Part model, mm, in its own coordinate system. A direction names the side the tool comes from. Give positions to 0.01 mm unless a question says otherwise; leave off trailing zeros. Write each loop counter-clockwise with the first axis right and the second up, starting at its lowest first coordinate (ties: lowest second). Pieces come first, ordered by that corner, then holes.
Autodesk Inventor part; units mm, degrees
ref_plane "YZ Plane" through (0, 0, 0) normal (1, 0, 0) x (0, 1, 0)
ref_plane "XZ Plane" through (0, 0, 0) normal (0, 1, 0) x (-1, 0, 0)
ref_plane "XY Plane" through (0, 0, 0) normal (0, 0, 1) x (1, 0, 0)
sketch "Sketch1" plane through (0, 0, 0) normal (0, 0, 1) x (1, 0, 0)
  line L0 (0, 0) -> (40, 0)
  line L1 (40, 0) -> (40, -40.5)
  line L2 (40, -40.5) -> (0, -40.5)
  line L3 (0, -40.5) -> (0, 0)
  dimension "d0" = 40
  dimension "d1" = 40.5
extrude "Extrusion1" add sketch "Sketch1" along normal mid plane 20
sketch "Sketch2" plane through (0, -40.5, 10) normal (-1, 0, 0) x (0, 0, 1)
  line L0 (0, 0) -> (-20, 0)
  line L1 (-20, 0) -> (-20, 40.5)
  line L2 (0, 40.5) -> (0, 0)
  circle A0 centre (-10, 10) radius 6
  line L3 (-20, 20.25) -> (0, 20.25)
  circle A1 centre (-10, 30.5) radius 6
  point P0 (-10, 40.5)
  dimension "d4" = 12
  dimension "d5" = 10
  dimension "d6" = 10
extrude "Extrusion2" add sketch "Sketch2" along normal blind 1.5 contours A0
sketch "Sketch3" plane through (40, -40.5, 10) normal (1, 0, 0) x (0, 0, -1)
  circle A0 centre (10, 10) radius 6
  circle A1 centre (10, 10) radius 6
  line L0 (0, 40.5) -> (0, 0)
  line L1 (0, 20.25) -> (20, 20.25)
  line L2 (20, 0) -> (20, 40.5)
  circle A2 centre (10, 30.5) radius 6
  point P0 (10, 40.5)
extrude "Extrusion4" add sketch "Sketch3" along normal blind 1.5 contours A0
extrude "Extrusion5" add sketch "Sketch2" along normal blind 0.1 contours A1
extrude "Extrusion6" add sketch "Sketch3" along normal blind 0.1 contours A2
properties part number "Motor"
1) Saw through at D-D (z = 8.75). Write the cut outline in (x, y), and give its area (3 significant figures).
Check result:
outline: (0, -40.5) - (40, -40.5) - (40, 0) - (0, 0) - close
area: 1,620 mm2
2) 3-axis set-ups, long thin cutter, end or side, ignore diameter. For faces 4 (the flat face through (41.5, -30, 0)), 5 (the cylindrical face through (40.74, -24.643, 1.301)), 6 (the flat face through (-0.1, -10, 0)), 7 (the flat face through (0, -21, 0)), 8 (the flat face through (20, -20, -10)): which of +Z, -Z, +X, -X, +Y, -Y reach the whole face in a straight line?
Check result:
face 4: +Z, -Z, +X, +Y, -Y
face 5: +X
face 6: +Z, -Z, -X, +Y
face 7: -X
face 8: -Z, +X, -X, +Y, -Y
3) Flat gauge pin, fed straight in: P1, Ø9.5, axis at y = -8.5, z = 2, coming from the -X side. Where does the tip first touch, or does it go through?
Check result:
P1: stops at x = -0.1
4) Saw through at B-B (z = 0). Write the cut outline in (x, y), and give its area (3 significant figures).
Check result:
outline: (-1.5, -36.5) - (0, -36.5) - (0, -40.5) - (40, -40.5) - (40, -36.5) - (41.5, -36.5) - (41.5, -24.5) - (40, -24.5) - (40, -16) - (40.1, -16) - (40.1, -4) - (40, -4) - (40, 0) - (0, 0) - (0, -4) - (-0.1, -4) - (-0.1, -16) - (0, -16) - (0, -24.5) - (-1.5, -24.5) - close
area: 1,660 mm2
5) Saw through at C-C (y = -10). Write the cut outline in (x, z).
Check result:
outline: (-0.1, -6) - (0, -6) - (0, -10) - (40, -10) - (40, -6) - (40.1, -6) - (40.1, 6) - (40, 6) - (40, 10) - (0, 10) - (0, 6) - (-0.1, 6) - close
6) Drill centre lines: L1, parallel to X at y = -9.5, z = 6.75; L2, parallel to X at y = -7, z = 2. Where is each one in solid material? Low to high.
Check result:
L1: x = 0 to 40
L2: x = -0.1 to 40.1
7) Mould opens along Y. For faces 1 (the flat face through (40, -20, 0)), 2 (the flat face through (40.1, -10, 0)), 3 (the flat face through (20, 0, 0)) say: +Y half, -Y half, draft (parallel to the pull), parting line (faces both ways), or undercut.
Check result:
face 1: undercut
face 2: draft
face 3: +Y half
8) Saw through at A-A (y = -30.5). Write the cut outline in (x, z), and give its area (3 significant figures).
Check result:
outline: (-1.5, -6) - (0, -6) - (0, -10) - (40, -10) - (40, -6) - (41.5, -6) - (41.5, 6) - (40, 6) - (40, 10) - (0, 10) - (0, 6) - (-1.5, 6) - close
area: 836 mm2
